The model under review builds one solid part; all positions refer to its coordinate system, in mm. Face numbers are marked on the shaded views. A direction names the side the tool comes from. Give positions to 0.01 mm unless a question says otherwise; leave off trailing zeros. Write each loop counter-clockwise with the first axis right and the second up, starting at its lowest first coordinate (ties: lowest second). Pieces come first, ordered by that corner, then holes. Notation, with made-up numbers: (-24.75, 56) - (-15.75, 56) arc R21 cw to (-15.75, 67) - close; hole circle Ø2 at (42.5, 67). An arc over 180 degrees is marked (long way). One line per question, with ' | ' between items. Start each with the question number.
```python
from build123d import *

# Parameters (mm, degrees)
CYLINDER011_R     = 2.5
CYLINDER011_DEPTH = 7.5
CYLINDER010_R     = 2.5
CYLINDER010_DEPTH = 7.5
EXTRUDE_DEPTH     = 4


with BuildPart() as cilindro010:
    # Cylinder011 → Cylinder011 (new body)
    with BuildSketch(Plane(origin=(27.5, 12, 5), x_dir=(1, 0, 0), z_dir=(0, 0, 1))):
        Circle(CYLINDER011_R)
    extrude(amount=CYLINDER011_DEPTH)


with BuildPart() as fusion002:
    # Cylinder010 → Cylinder010 (new body)
    with BuildSketch(Plane(origin=(-27.5, 12, 5), x_dir=(1, 0, 0), z_dir=(0, 0, 1))):
        Circle(CYLINDER010_R)
    extrude(amount=CYLINDER010_DEPTH)

    # Fusion002: union Cilindro010
    add(cilindro010.part)


with BuildPart() as obj1:
    # Sketch003 (on Face2 of Cylinder008) → Extrude (new body)
    with BuildSketch(Plane(origin=(0, 12, 1.5), x_dir=(1, 0, 0), z_dir=(0, 0, 1))):
        with BuildLine():
            Line((-23.5, 0), (-23.5, 11.330372))
            ThreePointArc((-18.962486, 15.867886), (-22.170993, 14.538879), (-23.5, 11.330372))
            Line((-18.962486, 15.867886), (18.940419, 15.867886))
            ThreePointArc((23.5, 11.308305), (22.16453, 14.532416), (18.940419, 15.867886))
            Line((23.5, 11.308305), (23.5, 0))
            ThreePointArc((23.5, 0), (27.5, -4), (31.5, 0))
            Line((31.5, 0), (31.5, 16.785542))
            ThreePointArc((31.5, 16.785542), (29.425629, 21.793515), (24.417656, 23.867886))
            Line((24.417656, 23.867886), (-21.265535, 23.867886))
            ThreePointArc((-21.265535, 23.867886), (-28.502395, 20.870281), (-31.5, 13.633421))
            Line((-31.5, 13.633421), (-31.5, 0))
            ThreePointArc((-31.5, 0), (-27.5, -4), (-23.5, 0))
        make_face()
    extrude(amount=EXTRUDE_DEPTH)


with BuildPart() as obj1_1:
    # Extrude placement: moved
    add(obj1.part.moved(Location((0, 0, 5))))

    # Cut002: cut Fusion002
    add(fusion002.part, mode=Mode.SUBTRACT)


solid = obj1_1.part
```
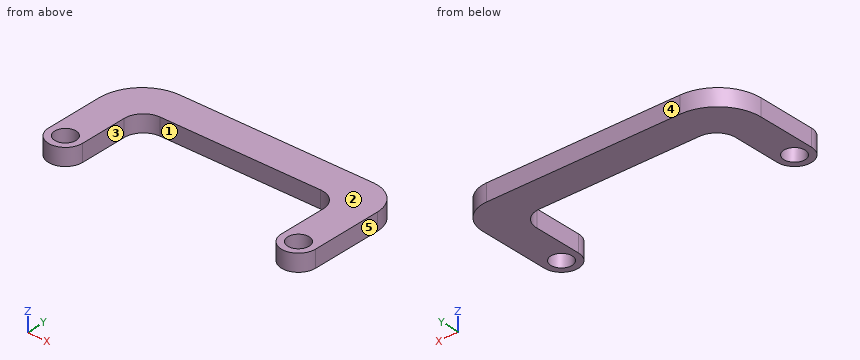
Item 1: Take a section at B-B (y = 15.25). Give the boundary of the cut face in (x, z), plus the area to 3 significant figures.
Item 2: Take a section at D-D (x = -14). Give the boundary of the cut face in (y, z).
Item 3: The part is to be moulded in two halves that separate along X. For the marked faces 3, 4 and 5, say which applies: +X half, -X half, draft (parallel to the pull), parting line (faces both ways), or undercut.
Item 4: Take a section at A-A (z = 8.3). Give the boundary of the cut face in (x, y), plus the area to 3 significant figures.
Item 5: Take a section at C-C (x = -27.5). Give the boundary of the cut face in (y, z).
Item 6: Machinability: for the marked faces 1 and 2, which of the approach directions +Z, -Z, +X, -X, +Y, -Y give a long, thin tool a straight path to every point of the face, cutting with its end or side? Answer none if there is none.
Item 7: Clearance check with flat-ended pins moving along their axes: P1, Ø3, axis at x = 27.5, y = 12, coming from the +Z side; P2, Ø1.5, axis at x = 9.5, z = 7, coming from the -Y side. State where each tip first meets the part, or that it passes through.
Item 8: For probe 1 along X at (y, z) = (12, 8.9); probe 2 along X at (y, z) = (21, 8.2); probe 3 along X at (y, z) = (13.75, 7.95), list the stretches that pass through material, from the lowest coordinate up.
Check sheet entries:
1) outline: (-31.5, 6.5) - (-23.5, 6.5) - (-23.5, 10.5) - (-31.5, 10.5) - close; (23.5, 6.5) - (31.5, 6.5) - (31.5, 10.5) - (23.5, 10.5) - close | area: 64.0 mm^2
2) outline: (27.87, 6.5) - (35.87, 6.5) - (35.87, 10.5) - (27.87, 10.5) - close
3) face 3: undercut | face 4: draft | face 5: +X half
4) outline: (-31.5, 12) arc R4 ccw to (-23.5, 12) - (-23.5, 23.33) arc R4.54 cw to (-18.96, 27.87) - (18.94, 27.87) arc R4.56 cw to (23.5, 23.31) - (23.5, 12) arc R4 ccw to (31.5, 12) - (31.5, 28.79) arc R7.08 ccw to (24.42, 35.87) - (-21.27, 35.87) arc R10.23 ccw to (-31.5, 25.63) - close; hole circle Ø5 at (-27.5, 12); hole circle Ø5 at (27.5, 12) | area: 745 mm^2
5) outline: (8, 6.5) - (9.5, 6.5) - (9.5, 10.5) - (8, 10.5) - close; (14.5, 6.5) - (33.75, 6.5) - (33.75, 10.5) - (14.5, 10.5) - close
6) face 1: +Z, -Z, -Y | face 2: +Z, +X, -X, +Y, -Y
7) P1: passes through | P2: stops at y = 27.87
8) probe 1: x = -31.5 to -30, -25 to -23.5, 23.5 to 25, 30 to 31.5 | probe 2: x = -31.5 to -23.5, 23.5 to 31.5 | probe 3: x = -31.5 to -29.29, -25.71 to -23.5, 23.5 to 25.71, 29.29 to 31.5
